```python
from build123d import *

# Parameters (mm, degrees)
F0_W     = 80
F0_H     = 80
F1_DEPTH = 25
F2_SIZE  = 30
F3_R     = 18.489641


with BuildPart() as f1:
    # F0 (on Right) → F1 (new body)
    with BuildSketch(Plane.YZ):
        with Locations((-9.415843, 26.514679)):
            Rectangle(F0_W, F0_H)
    extrude(amount=F1_DEPTH)

    # F2
    f2_edges = [f1.edges().sort_by_distance(p)[0] for p in [
        (12.5, 30.584157, 66.514679),
    ]]
    chamfer(f2_edges, length=F2_SIZE)

    # F3
    f3_edges = [f1.edges().sort_by_distance(p)[0] for p in [
        (25, -49.415843, 26.514679),
    ]]
    fillet(f3_edges, radius=F3_R)


solid = f1.part
```
Geometry check sheet. Reference: the model listing, model coordinates, mm. Round coordinates to 2 decimals unless told otherwise and drop trailing zeros. Write each loop counter-clockwise with the first axis right and the second up, starting at its lowest first coordinate (ties: lowest second). Pieces come first, ordered by that corner, then holes. Notation, with made-up numbers: (-35, 15.5) - (12, 15.5) arc R30 ccw to (12, 44.5) - close; hole circle Ø4 at (-9, -32.5). An arc over 180 degrees is marked (long way). Write each question's results on one line, items separated by ' | '.
(1) Thickness scan on probe 1 along Y at (x, z) = (16.25, -8); probe 2 along Z at (x, y) = (15.5, 17); probe 3 along Y at (x, z) = (22, 27). Record the ranges inside material, lowest first. Write a range as from..to.
Computed:
probe 1: y = -46.64..30.58 | probe 2: z = -13.49..50.1 | probe 3: y = -41.02..30.58
(2) Sectioned sample at C-C, the plane y = -42. Enter the section's corners in (x, z), plus the area to 3 significant figures.
Computed:
outline: (0, -13.49) - (21.32, -13.49) - (21.32, 66.51) - (0, 66.51) - close | area: 1,710 mm^2
(3) Depth check by flat-ended pin: pin 1 Ø8 at (x, z) = (14.5, 28.5) entering from -Y. Enter the tip coordinate at first touch or a pass-through.
Computed:
pin 1: stops at y = -48.98
(4) Sectioned sample at D-D, the plane y = 10. Enter the section's corners in (x, z).
Computed:
outline: (0, -13.49) - (25, -13.49) - (25, 57.1) - (0, 57.1) - close
(5) Sectioned sample at B-B, the plane x = 1.5. Enter the section's corners in (y, z).
Computed:
outline: (-49.42, -13.49) - (30.58, -13.49) - (30.58, 36.51) - (0.58, 66.51) - (-49.42, 66.51) - close
(6) Sectioned sample at A-A, the plane z = 31. Enter the section's corners in (x, y).
Computed:
outline: (0, -49.42) - (6.51, -49.42) arc R18.49 ccw to (25, -30.93) - (25, 30.58) - (0, 30.58) - close
